Geometry check sheet. Reference: the model listing, model coordinates, mm. Face numbers are marked on the shaded views. A direction names the side the tool comes from. Round coordinates to 2 decimals unless told otherwise and drop trailing zeros. Order: outer loops, then holes, each group sorted by start corner. A loop starts at its lowest first (then second) coordinate and runs counter-clockwise, first axis right, second up.
(1) Sectioned sample at A-A (z = 46). Record the boundary of the cut face in (x, y), plus the area to 3 significant figures.
(2) Go/stop test with flat-tipped pins: pin 1 (6 mm diameter, centred on x = 11.5, y = 21, fed in from +Z); pin 2 (24 mm diameter, centred on x = 10, z = 25, fed in from -Y); pin 3 (8 mm diameter, centred on x = 29.5, z = 19.5, fed in from -Y). Record where each tip stops, or that it passes through.
(3) Sectioned sample at C-C (x = 23). Record the boundary of the cut face in (y, z).
(4) Set-up check for the marked faces 1, 2 and 3: record each of +Z, -Z, +X, -X, +Y, -Y from which the full face is reachable in a straight line by a thin tool's end or side.
(5) Sectioned sample at B-B (y = 41.5). Record the boundary of the cut face in (x, z).
(6) Material ranges on line 1 along Y through (x, z) = (15, 32); line 2 along X through (y, z) = (13, 33); line 3 along Y through (x, z) = (47, 38), recorded low to high.
(7) Release check for a two-part mould opening along X. For the marked faces 4, 5, 6 and 7 record: +X half, -X half, draft (parallel to the pull), parting line (faces both ways), or undercut.
(8) Sectioned sample at D-D (z = 5.5). Record the boundary of the cut face in (x, y).
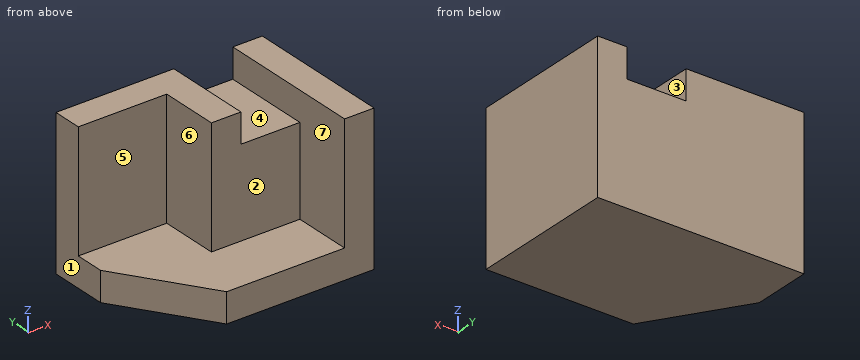
from build123d import *

# Parameters (mm, degrees)
SKETCH1_W           = 70
SKETCH1_H           = 50
BOSS_EXTRUDE1_DEPTH = 50
CUT_EXTRUDE2_DEPTH  = 50
CUT_EXTRUDE4_DEPTH  = 40
SKETCH5_W           = 20
SKETCH5_H           = 10
CUT_EXTRUDE5_DEPTH  = 40


with BuildPart() as part:
    # Sketch1 → Boss-Extrude1 (new body)
    with BuildSketch(Plane.XY):
        with Locations((35, 25)):
            Rectangle(SKETCH1_W, SKETCH1_H)
    extrude(amount=BOSS_EXTRUDE1_DEPTH)

    # Sketch3 → Cut-Extrude2 (cut)
    with BuildSketch(Plane.XY):
        Polygon((0, 30), (20, 0), (0, 0), align=None)
    extrude(amount=CUT_EXTRUDE2_DEPTH, mode=Mode.SUBTRACT)

    # Sketch4 → Cut-Extrude4 (cut)
    with BuildSketch(Plane.XY.offset(50)):
        Polygon((60, 0), (60, 20), (30, 20), (30, 40), (0, 40), (0, 30), (20, 0), align=None)
    extrude(amount=-CUT_EXTRUDE4_DEPTH, mode=Mode.SUBTRACT)

    # Sketch5 → Cut-Extrude5 (cut)
    with BuildSketch(Plane.XZ.offset(-20)):
        with Locations((50, 45)):
            Rectangle(SKETCH5_W, SKETCH5_H)
    extrude(amount=-CUT_EXTRUDE5_DEPTH, mode=Mode.SUBTRACT)


solid = part.part
Answer below:
1. outline: (0, 40) - (30, 40) - (30, 20) - (40, 20) - (40, 50) - (0, 50) - close; (60, 0) - (70, 0) - (70, 50) - (60, 50) - close
1. area: 1,100 mm2
2. pin 1: stops at z = 10
2. pin 2: stops at y = 40
2. pin 3: stops at y = 20
3. outline: (0, 0) - (50, 0) - (50, 50) - (40, 50) - (40, 10) - (0, 10) - close
4. face 1: +Z, -Z, -X, +Y, -Y
4. face 2: +Z, -X, -Y
4. face 3: +Z, +Y, -Y
5. outline: (0, 0) - (70, 0) - (70, 50) - (60, 50) - (60, 40) - (40, 40) - (40, 50) - (0, 50) - close
6. line 1: y = 40 to 50
6. line 2: x = 60 to 70
6. line 3: y = 20 to 50
7. face 4: undercut
7. face 5: draft
7. face 6: -X half
7. face 7: undercut
8. outline: (0, 30) - (20, 0) - (70, 0) - (70, 50) - (0, 50) - close
